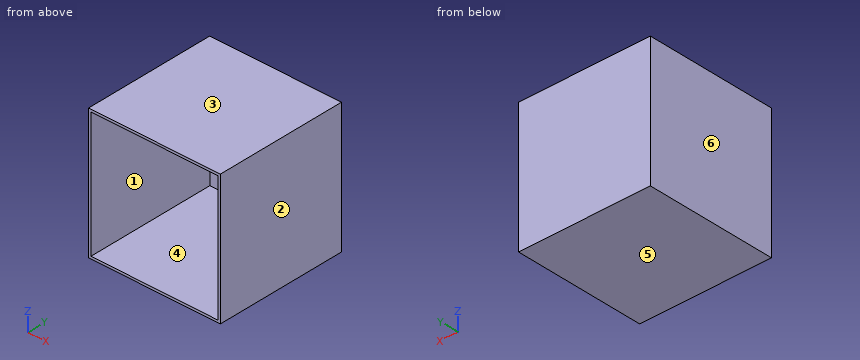
```python
from build123d import *

# Parameters (mm, degrees)
F0_W     = 550
F0_H     = 550
F1_DEPTH = 550
F2_W     = 530
F2_H     = 530
F3_DEPTH = 540


with BuildPart() as f1:
    # F0 (on Top) → F1 (new body)
    with BuildSketch(Plane.XY):
        with Locations((-236.357567, 253.178654)):
            Rectangle(F0_W, F0_H)
    extrude(amount=-F1_DEPTH)

    # F2 (on face) → F3 (cut)
    with BuildSketch(Plane.XZ.offset(21.821346)):
        with Locations((-236.357567, -275)):
            Rectangle(F2_W, F2_H)
    extrude(amount=-F3_DEPTH, mode=Mode.SUBTRACT)


solid = f1.part
```
The model under review builds one solid part; all positions refer to its coordinate system, in mm. Face numbers are marked on the shaded views. A direction names the side the tool comes from. Round coordinates to 2 decimals unless told otherwise and drop trailing zeros. Write each loop counter-clockwise with the first axis right and the second up, starting at its lowest first coordinate (ties: lowest second). Pieces come first, ordered by that corner, then holes. Notation, with made-up numbers: (27.5, 47) -> (46.5, 47) arc R24 ccw to (46.5, 71) -> close; hole circle Ø2 at (15, -11). An arc over 180 degrees is marked (long way). Use CSV: the item, a comma, the result in double quotes.
Q1. To check wall thickness, follow probe 1 along Z at (x, y) = (-53, 287.5); probe 2 along X at (y, z) = (165, -421); probe 3 along Y at (x, z) = (-178.5, -71). State the ranges of each line that lie inside material, in increasing order. Write a range as [from, to].
Checks:
probe 1,"[-550, -540], [-10, 0]"
probe 2,"[-511.36, -501.36], [28.64, 38.64]"
probe 3,"[518.18, 528.18]"
Q2. For the marked faces 1 and 2, list the 3-axis set-ups (+Z, -Z, +X, -X, +Y, -Y) from which the entire face can be reached by the end or side of a thin tool; tool diameter is ignored.
Checks:
face 1,"-Y"
face 2,"+Z, -Z, +X, +Y, -Y"
Q3. Consider section B-B (z = -427). Give the boundary of the cut face in (x, y).
Checks:
outline,"(-511.36, -21.82) -> (-501.36, -21.82) -> (-501.36, 518.18) -> (28.64, 518.18) -> (28.64, -21.82) -> (38.64, -21.82) -> (38.64, 528.18) -> (-511.36, 528.18) -> close"
Q4. For pin 1 Ø1.5 at (x, z) = (-118, -332.5) entering from -Y, flat-tipped, find the tip position at first contact; note if it passes through.
Checks:
pin 1,"y = 518.18"
Q5. Consider section C-C (x = -345). Give the boundary of the cut face in (y, z), then the cut area to 3 significant figures.
Checks:
outline,"(-21.82, -550) -> (528.18, -550) -> (528.18, 0) -> (-21.82, 0) -> (-21.82, -10) -> (518.18, -10) -> (518.18, -540) -> (-21.82, -540) -> close"
area,"16,300 mm²"
Q6. Consider section A-A (y = 310). Give the boundary of the cut face in (x, z), then the cut area to 3 significant figures.
Checks:
outline,"(-511.36, -550) -> (38.64, -550) -> (38.64, 0) -> (-511.36, 0) -> close; hole (-501.36, -540) -> (28.64, -540) -> (28.64, -10) -> (-501.36, -10) -> close"
area,"21,600 mm²"
Q7. Mouldability with a two-part tool opening along Z and no side actions: class the marked faces 3, 4, 5 and 6 as released by +Z, released by -Z, zero draft, split by the parting line, or undercut.
Checks:
face 3,"released by +Z"
face 4,"undercut"
face 5,"released by -Z"
face 6,"zero draft"
